The model under review builds one solid part; all positions refer to its coordinate system, in mm. A direction names the side the tool comes from. Round coordinates to 2 decimals unless told otherwise and drop trailing zeros. Use CSV: the item, a comma, the result in double quotes. Start each with the question number.
1) Mouldability with a two-part tool opening along Z and no side actions: class faces 4 (the face through (-0.1, 0.5, 61.9)), 5 (the face through (-61.924, -0.166, 0.526)), 6 (the face through (3.03, -0.95, 69.94)) as released by +Z, released by -Z, zero draft, split by the parting line, or undercut.
2) Wall thickness on probe 1 along Z at (x, y) = (73.75, 0) (3 decimals); probe 2 along Y at (x, z) = (0, 67) (1 decimal): over which ranges is each line inside the solid? List them lowest first. Write a range as [from, to].
3) Machinability: for faces 1 (the face through (-1.5, 2.8, -69.9)), 2 (the face through (69.94, 3.1, 0.69)), 3 (the face through (-69.94, -0.95, 3.03)), which of the approach directions +Z, -Z, +X, -X, +Y, -Y give a long, thin tool a straight path to every point of the face, cutting with its end or side? Answer none if there is none.
4) For pin 1 Ø5 at (x, y) = (0, 0) entering from +Z, flat-tipped, find the tip position at first contact; note if it passes through.
from build123d import *

# Parameters (mm, degrees)
SKETCH1_W           = 152.4
SKETCH1_H           = 152.4
BOSS_EXTRUDE1_DEPTH = 4.7625
CIRPATTERN1_COUNT   = 4


with BuildPart() as part:
    # Sketch1 → Boss-Extrude1 (new, symmetric)
    with BuildSketch(Plane(origin=(0, 0, 0), x_dir=(1, 0, 0), z_dir=(0, 1, 0))):
        Rectangle(SKETCH1_W, SKETCH1_H)
    extrude(amount=BOSS_EXTRUDE1_DEPTH, both=True)

    # Sketch3 → 1_4 _0.25_ Diameter Hole1 (revolve, cut)
    with BuildSketch(Plane(origin=(76.2, 0, 0), x_dir=(0, 0, -1), z_dir=(0, 1, 0))):
        Polygon((0, 0), (0, 14.607732465), (3.175, 12.7), (3.175, 0), align=None)
    f_1_4_0_25_diameter_hole1 = revolve(axis=Axis((82.55, 0, 0), (-1, 0, 0)), mode=Mode.SUBTRACT)

    # CirPattern1: 1_4 _0.25_ Diameter Hole1 ×4 about axis
    cirpattern1_axis = Axis((0, 4.7625, 0), (0, -1, 0))
    for i in range(1, CIRPATTERN1_COUNT):
        add(f_1_4_0_25_diameter_hole1.rotate(cirpattern1_axis, i * 360 / CIRPATTERN1_COUNT), mode=Mode.SUBTRACT)


solid = part.part
Values found:
1,face 4,"released by +Z"
1,face 5,"undercut"
1,face 6,"zero draft"
2,probe 1,"[-76.2, -3.175], [3.175, 76.2]"
2,probe 2,"[-4.8, -3.2], [3.2, 4.8]"
3,face 1,"-Z"
3,face 2,"+X"
3,face 3,"-X"
4,pin 1,"z = 63.09"
